Can you work these out from the model? Positions are in its coordinate system, mm. A direction names the side the tool comes from. Give positions to 0.01 mm unless a question says otherwise; leave off trailing zeros. Write each loop counter-clockwise with the first axis right and the second up, starting at its lowest first coordinate (ties: lowest second). Pieces come first, ordered by that corner, then holes. Notation, with made-up numbers: M 25,48 L 66,48 A9 ccw 66,52 Z; hole C 19.25,-2.5 d1. An arc over 180 degrees is marked long. Use CSV: the item, a comma, the result in double quotes. Start each with the question number.
from build123d import *

# Parameters (mm, degrees)
SKETCH1_R                = 99.06
BOSS_EXTRUDE1_DEPTH      = 35.56
BOSS_EXTRUDE1_DEPTH_BACK = 35.56
SKETCH3_OUTSIDE_W        = 257.934
SKETCH3_OUTSIDE_H        = 257.934
SKETCH3_OUTSIDE_R        = 41.91
CUT_EXTRUDE1_DEPTH       = 27.94
CUT_EXTRUDE1_DEPTH_BACK  = 27.94
SKETCH4_R                = 12.7
CUT_EXTRUDE2_DEPTH       = 36.56
CUT_EXTRUDE2_DEPTH_BACK  = 36.56


with BuildPart() as part:
    # Sketch1 → Boss-Extrude1 (new body, two sides)
    with BuildSketch(Plane.XY) as boss_extrude1_sk:
        Circle(SKETCH1_R)
    extrude(amount=BOSS_EXTRUDE1_DEPTH)
    extrude(boss_extrude1_sk.sketch, amount=-BOSS_EXTRUDE1_DEPTH_BACK)

    # Sketch3 outside → Cut-Extrude1 (cut, two sides)
    with BuildSketch(Plane.XY) as cut_extrude1_sk:
        Rectangle(SKETCH3_OUTSIDE_W, SKETCH3_OUTSIDE_H)
        Circle(SKETCH3_OUTSIDE_R, mode=Mode.SUBTRACT)
    extrude(amount=CUT_EXTRUDE1_DEPTH, mode=Mode.SUBTRACT)
    extrude(cut_extrude1_sk.sketch, amount=-CUT_EXTRUDE1_DEPTH_BACK, mode=Mode.SUBTRACT)

    # Sketch4 → Cut-Extrude2 (cut, two sides)
    with BuildSketch(Plane.XY) as cut_extrude2_sk:
        Circle(SKETCH4_R)
    extrude(amount=CUT_EXTRUDE2_DEPTH, mode=Mode.SUBTRACT)
    extrude(cut_extrude2_sk.sketch, amount=-CUT_EXTRUDE2_DEPTH_BACK, mode=Mode.SUBTRACT)


solid = part.part
(1) Thinking about a two-plate mould opening in Z: for faces 3 (the face through (94.486, 29.755, 31.803)), 4 (the face through (21, 1, 35.56)), 5 (the face through (-5.456, 41.553, 0.391)), which applies, released by +Z, released by -Z, zero draft, split by the parting line, or undercut?
(2) I want a section at A-A (x = 0). Write out the boundary of the cut face in (y, z).
(3) I want a section at B-B (y = 63). Write out the boundary of the cut face in (x, z).
(4) Please list where these lines run through material, in increasing order: L1, parallel to Z at x = 54, y = -78.5; L2, parallel to Y at x = 0, z = 7; L3, parallel to Y at x = -4, z = -2.5. Write a range as [from, to].
(5) Which directions (+Z, -Z, +X, -X, +Y, -Y) give clear straight access to the entire face, cutting with the end or side of a thin tool? Please do faces 1 (the face through (43, 1, -27.94)), 2 (the face through (-2.75, -12.4, 0.5)).
(6) Will these pins go through, and if not, where does the flat tip stop? pin 1 Ø1 at (x, z) = (33.5, 14) entering from -Y (3 decimals); pin 2 Ø12 at (y, z) = (-66.5, -27) entering from +X; pin 3 Ø6 at (x, z) = (-59, 24.5) entering from +Y; pin 4 Ø10 at (x, z) = (-32.5, -14.5) entering from -Y.
(7) I want a section at C-C (z = 21). Write out the boundary of the cut face in (x, y).
Geometry results:
1,face 3,"zero draft"
1,face 4,"released by +Z"
1,face 5,"undercut"
2,outline,"M -99.06,-35.56 L -12.7,-35.56 L -12.7,35.56 L -99.06,35.56 L -99.06,27.94 L -41.91,27.94 L -41.91,-27.94 L -99.06,-27.94 Z; M 12.7,-35.56 L 99.06,-35.56 L 99.06,-27.94 L 41.91,-27.94 L 41.91,27.94 L 99.06,27.94 L 99.06,35.56 L 12.7,35.56 Z"
3,outline,"M -76.45,-35.56 L 76.45,-35.56 L 76.45,-27.94 L -76.45,-27.94 Z; M -76.45,27.94 L 76.45,27.94 L 76.45,35.56 L -76.45,35.56 Z"
4,L1,"z = [-35.56, -27.94], [27.94, 35.56]"
4,L2,"y = [-41.91, -12.7], [12.7, 41.91]"
4,L3,"y = [-41.72, -12.05], [12.05, 41.72]"
5,face 1,"none"
5,face 2,"+Z, -Z"
6,pin 1,"stops at y = -25.835"
6,pin 2,"stops at x = 78.38"
6,pin 3,"passes through"
6,pin 4,"stops at y = -31.63"
7,outline,"C 0,0 d83.82; hole C 0,0 d25.4"
